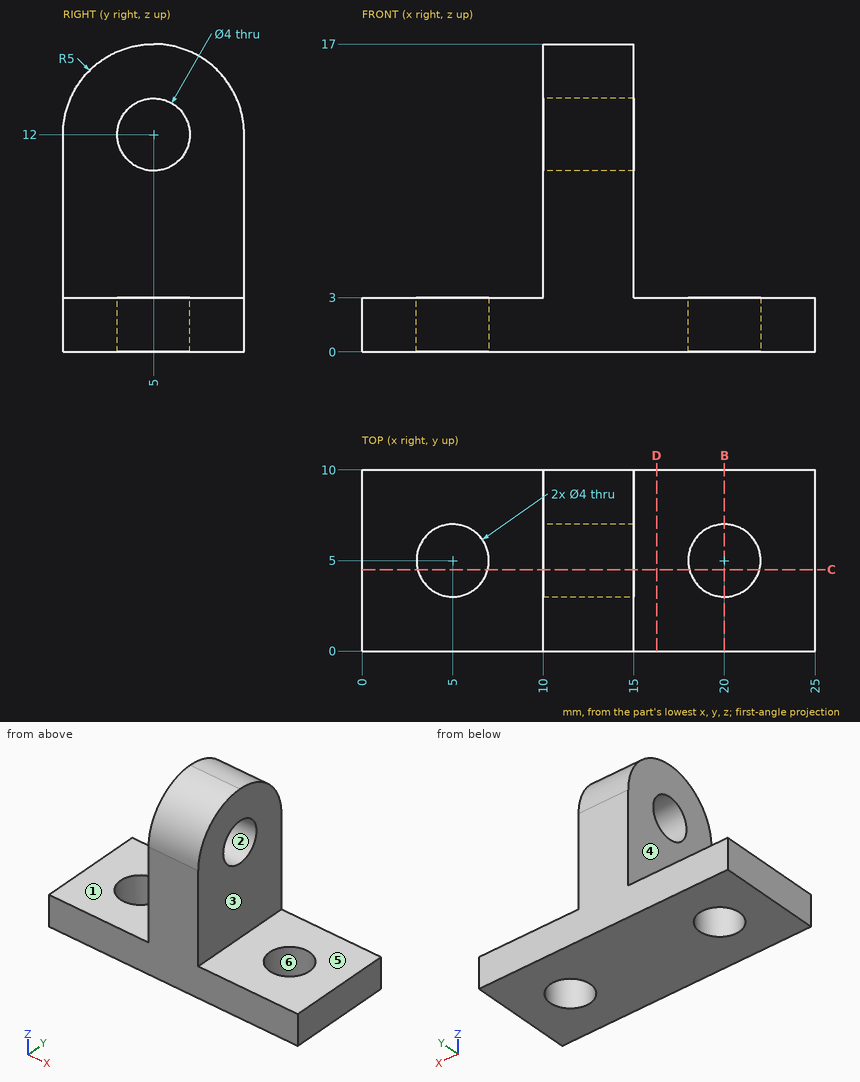
Study the drawing (mm; zero at the part's minimum x, y, z) and answer. A direction names the side the tool comes from. Coordinates: 2 decimals unless noted, no trailing zeros. Order: outer loops, then holes, each group sorted by start corner. A loop starts at its lowest first (then second) coordinate and runs counter-clockwise, first axis right, second up. Notation, with made-up numbers: M 21,51.25 L 70,51.25 A19 ccw 70,61.25 Z; hole C 47,50.25 d7. An arc over 180 degrees is marked long. Use CSV: the item, a comma, the result in double quotes.
Q1. Section C-C (y = 4.5) is taken. Determine the outline of the cut face in (x, z), then the cut area to 3 significant figures.
Here are the results:
outline,"M 0,0 L 3.06,0 L 3.06,3 L 0,3 Z; M 6.94,0 L 18.06,0 L 18.06,3 L 15,3 L 15,10.06 L 10,10.06 L 10,3 L 6.94,3 Z; M 10,13.94 L 15,13.94 L 15,16.97 L 10,16.97 Z; M 21.94,0 L 25,0 L 25,3 L 21.94,3 Z"
area,"102 mm2"
Q2. Section D-D (x = 16.25) is taken. Determine the outline of the cut face in (y, z), then the cut area to 3 significant figures.
Here are the results:
outline,"M 0,0 L 10,0 L 10,3 L 0,3 Z"
area,"30.0 mm2"
Q3. Given pin 1 Ø3 at (y, z) = (5, 11) entering from -X; pin 2 Ø5 at (y, z) = (7.5, 6.5) entering from +X, each flat-ended and moving along its own axis, determine where each tip first touches the part or whether it passes through.
Here are the results:
pin 1,"x = 10"
pin 2,"x = 15"
Q4. Section B-B (x = 20) is taken. Determine the outline of the cut face in (y, z).
Here are the results:
outline,"M 0,0 L 3,0 L 3,3 L 0,3 Z; M 7,0 L 10,0 L 10,3 L 7,3 Z"
Q5. Determine the mould class of the marked faces 4, 5 and 6 for opening direction X: pulls with the +X half, pulls with the -X half, needs draft (parallel to the pull), parting line crosses it, or undercut.
Here are the results:
face 4,"pulls with the -X half"
face 5,"needs draft"
face 6,"undercut"
Q6. A tool of negligible diameter and unlimited length cuts with its end or side. For the marked faces 1, 2 and 3, from which of +Z, -Z, +X, -X, +Y, -Y can it reach the whole face along a straight path? Write none if from no direction.
Here are the results:
face 1,"+Z, -X, +Y, -Y"
face 2,"+X, -X"
face 3,"+Z, +X, +Y, -Y"
Q7. Straight lines are drawn through the part: L1, parallel to Y at x = 5, z = 0.6; L2, parallel to X at y = 9.75, z = 13.25; L3, parallel to Z at x = 8.25, y = 6.5. For each, find the intervals that lie inside material, in ascending order.
Here are the results:
L1,"0 to 3, 7 to 10"
L2,"10 to 15"
L3,"0 to 3"
